```python
from build123d import *

# Parameters (mm, degrees)
SKETCH1_W                       = 9
SKETCH1_H                       = 18
SKETCH1_R                       = 1.9
BODY_MOUNT_DEPTH                = 3
SKETCH2_W                       = 5
SKETCH2_H                       = 3
BOSS_EXTRUDE2_DEPTH             = 25
SKETCH3_W                       = 5
SKETCH3_H                       = 5
BOSS_EXTRUDE3_DEPTH             = 20
SKETCH4_R                       = 1.5
CUT_EXTRUDE1_DEPTH              = 20
BOSS_EXTRUDE4_REACH             = 38.359
BOSS_EXTRUDE4_DIRECTION_2_REACH = 38.359
FILLET2_R                       = 5


with BuildPart() as part:
    # Sketch1 → body mount (new body)
    with BuildSketch(Plane(origin=(0, 0, 0), x_dir=(1, 0, 0), z_dir=(0, 1, 0))):
        with Locations((-0.5, 5)):
            Rectangle(SKETCH1_W, SKETCH1_H)
        with Locations(Location((0, 0, 0), (0, 0, 270))):
            Circle(SKETCH1_R, mode=Mode.SUBTRACT)
        with Locations(Location((0, 10, 0), (0, 0, 270))):
            Circle(SKETCH1_R, mode=Mode.SUBTRACT)
    extrude(amount=BODY_MOUNT_DEPTH)

    # Sketch2 → Boss-Extrude2 (add)
    with BuildSketch(Plane(origin=(4, 0, 0), x_dir=(0, 0, -1), z_dir=(1, 0, 0))):
        with Locations((5, 1.5)):
            Rectangle(SKETCH2_W, SKETCH2_H)
    extrude(amount=BOSS_EXTRUDE2_DEPTH)

    # Sketch3 → Boss-Extrude3 (add)
    with BuildSketch(Plane.XZ):
        with Locations((26.5, -5)):
            Rectangle(SKETCH3_W, SKETCH3_H)
    extrude(amount=BOSS_EXTRUDE3_DEPTH)

    # Sketch4 → Cut-Extrude1 (cut)
    with BuildSketch(Plane(origin=(0, 0, -7.5), x_dir=(-1, 0, 0), z_dir=(0, 0, -1))):
        with Locations((-26.5, -17)):
            Circle(SKETCH4_R)
        with Locations((-26.5, -7.5)):
            Circle(SKETCH4_R)
    extrude(amount=-CUT_EXTRUDE1_DEPTH, mode=Mode.SUBTRACT)

    # Boss-Extrude4: up to this face of the body (flat: up to its plane)
    boss_extrude4_end = Plane(part.part.faces().sort_by_distance((16.5, 2.660294245, -7.5))[0])
    # Sketch5 → Boss-Extrude4 (add, up to the picked face)
    with BuildSketch(Plane(origin=(0, 0, -5), x_dir=(-1, 0, 0), z_dir=(0, 0, -1)), mode=Mode.PRIVATE) as boss_extrude4_sk1:
        Polygon((-24, -10.415369352), (-9.210305315, 0), (-4, 0), (-24, -14.084630648), align=None)
    boss_extrude4_tool1 = split(extrude(boss_extrude4_sk1.sketch, amount=BOSS_EXTRUDE4_REACH, mode=Mode.PRIVATE), bisect_by=boss_extrude4_end, keep=Keep.BOTH, mode=Mode.PRIVATE)
    add(boss_extrude4_tool1.solids().sort_by(Axis((15.237549, -6.170794, -5), (0, 0, -1)))[0])

    # Boss-Extrude4 direction 2: up to this face of the body (flat: up to its plane)
    boss_extrude4_direction_2_end = Plane(part.part.faces().sort_by_distance((14, 0.339705755, -2.5))[0])
    # Sketch5 → Boss-Extrude4 direction 2 (add, up to the picked face)
    with BuildSketch(Plane(origin=(0, 0, -5), x_dir=(-1, 0, 0), z_dir=(0, 0, -1)), mode=Mode.PRIVATE) as boss_extrude4_direction_2_sk1:
        Polygon((-24, -10.415369352), (-9.210305315, 0), (-4, 0), (-24, -14.084630648), align=None)
    boss_extrude4_direction_2_tool1 = split(extrude(boss_extrude4_direction_2_sk1.sketch, amount=-BOSS_EXTRUDE4_DIRECTION_2_REACH, mode=Mode.PRIVATE), bisect_by=boss_extrude4_direction_2_end, keep=Keep.BOTH, mode=Mode.PRIVATE)
    add(boss_extrude4_direction_2_tool1.solids().sort_by(Axis((15.237549, -6.170794, -5), (0, 0, 1)))[0])

    # Fillet2
    # the kernel refuses this fillet: 5 mm, written as the material it adds along each edge
    with BuildSketch(Plane(origin=(4, 3, -7.5), x_dir=(0, 0, -1), z_dir=(0, -1, 0))) as fillet2_piece_1_section:
        with BuildLine():
            CenterArc((FILLET2_R, FILLET2_R), FILLET2_R, 180, 90)
            Line((0, FILLET2_R), (0, 0))
            Line((0, 0), (FILLET2_R, 0))
        make_face()
    fillet2_piece_1 = extrude(amount=3, mode=Mode.PRIVATE)
    fillet2_piece_1 = split(fillet2_piece_1, bisect_by=Plane(origin=(4.050655402, -0.035673131, -8.630736825), z_dir=(0.5757819971310116, 0.8176032606220598, 0)), keep=Keep.TOP, mode=Mode.PRIVATE)
    add(fillet2_piece_1)
    with BuildSketch(Plane(origin=(4, 3, -7.5), x_dir=(0, 0, -1), z_dir=(0, -1, 0))) as fillet2_piece_2_section:
        with BuildLine():
            CenterArc((FILLET2_R, FILLET2_R), FILLET2_R, 180, 90)
            Line((0, FILLET2_R), (0, 0))
            Line((0, 0), (FILLET2_R, 0))
        make_face()
    fillet2_piece_2 = extrude(amount=15.5, mode=Mode.PRIVATE)
    fillet2_piece_2 = split(fillet2_piece_2, bisect_by=Plane(origin=(6.150590259, 0, -8.032362576), z_dir=(0, -1, 0)), keep=Keep.TOP, mode=Mode.PRIVATE)
    fillet2_piece_2 = split(fillet2_piece_2, bisect_by=Plane(origin=(5.79410314, -1.263464003, -8.032362576), z_dir=(0.5757819971310116, 0.8176032606220598, 0)), keep=Keep.TOP, mode=Mode.PRIVATE)
    add(fillet2_piece_2)
    with BuildSketch(Plane(origin=(4, -12.5, -2.5), x_dir=(1, 0, 0), z_dir=(0, 1, 0))) as fillet2_piece_3_section:
        with BuildLine():
            CenterArc((FILLET2_R, -FILLET2_R), FILLET2_R, 90, 90)
            Line((0, -FILLET2_R), (0, 0))
            Line((0, 0), (FILLET2_R, 0))
        make_face()
    fillet2_piece_3 = extrude(amount=15.5, mode=Mode.PRIVATE)
    fillet2_piece_3 = split(fillet2_piece_3, bisect_by=Plane(origin=(5.79410314, -1.263464003, -1.967637424), z_dir=(0.5757819971310116, 0.8176032606220598, 0)), keep=Keep.TOP, mode=Mode.PRIVATE)
    fillet2_piece_3 = split(fillet2_piece_3, bisect_by=Plane(origin=(6.150590259, 0, -1.967637424), z_dir=(0, -1, 0)), keep=Keep.TOP, mode=Mode.PRIVATE)
    add(fillet2_piece_3)
    with BuildSketch(Plane(origin=(4, 0, -2.5), x_dir=(1, 0, 0), z_dir=(0, 1, 0))) as fillet2_piece_4_section:
        with BuildLine():
            CenterArc((FILLET2_R, -FILLET2_R), FILLET2_R, 90, 90)
            Line((0, -FILLET2_R), (0, 0))
            Line((0, 0), (FILLET2_R, 0))
        make_face()
    fillet2_piece_4 = extrude(amount=3, mode=Mode.PRIVATE)
    fillet2_piece_4 = split(fillet2_piece_4, bisect_by=Plane(origin=(4.050655402, -0.035673131, -1.369263175), z_dir=(0.5757819971310116, 0.8176032606220598, 0)), keep=Keep.TOP, mode=Mode.PRIVATE)
    add(fillet2_piece_4)


solid = part.part
```
CAD build for the part. Positions are in the model's coordinates, mm. A direction names the side the tool comes from. Coordinates: 2 decimals unless noted, no trailing zeros. Order: outer loops, then holes, each group sorted by start corner. A loop starts at its lowest first (then second) coordinate and runs counter-clockwise, first axis right, second up. Notation, with made-up numbers: M 43.5,28.5 L 88.5,28.5 A23 cw 88.5,45.5 Z; hole C 1.5,49 d3. An arc over 180 degrees is marked long. Answer as CSV lines item,"result".
1) Cut at A-A (x = 0). List the corners of the cut face in (y, z).
Verdict:
outline,"M 0,-14 L 3,-14 L 3,-11.9 L 0,-11.9 Z; M 0,-8.1 L 3,-8.1 L 3,-1.9 L 0,-1.9 Z; M 0,1.9 L 3,1.9 L 3,4 L 0,4 Z"
2) Flat gauge pins, fed straight in: P1, Ø1.2, axis at y = 1.5, z = -13, coming from the +X side; P2, Ø5, axis at x = 26.5, y = -17, coming from the -Z side; P3, Ø1.5, axis at y = -18.5, z = -6, coming from the -X side. Where does each tip first touch, or does it go through?
Verdict:
P1,"x = 4"
P2,"z = -7.5"
P3,"x = 24"
3) Mould opens along X. For faces 1 (the flat face through (26, -20, -5)), 2 (the cylindrical face through (6.18, 0.42, -1.63)), 3 (the flat face through (24, -5, -5)), 4 (the flat face through (24, -17, -5)) say: released by +X, released by -X, zero draft, split by the parting line, or undercut.
Verdict:
face 1,"zero draft"
face 2,"released by +X"
face 3,"undercut"
face 4,"released by -X"
4) Cut at B-B (y = -17). List the corners of the cut face in (x, z), then the cut area to 3 significant figures.
Verdict:
outline,"M 24,-7.5 L 25,-7.5 L 25,-2.5 L 24,-2.5 Z; M 28,-7.5 L 29,-7.5 L 29,-2.5 L 28,-2.5 Z"
area,"10.0 mm2"
5) 3-axis set-ups, long thin cutter, end or side, ignore diameter. For faces 5 (the flat face through (4, 1, 3)), 6 (the flat face through (8, 3, -5)), 7 (the flat face through (21, -9, -7.5)), 8 (the flat face through (17, 0, -5)), 9 (the flat face through (-5, 1, -5)): which of +Z, -Z, +X, -X, +Y, -Y reach the whole face in a straight line?
Verdict:
face 5,"+Z, +X, +Y, -Y"
face 6,"+Z, -Z, +X, -X, +Y"
face 7,"-Z, +X, +Y, -Y"
face 8,"+Z, -Z"
face 9,"+Z, -Z, -X, +Y, -Y"
6) Cut at D-D (y = 1). List the corners of the cut face in (x, z).
Verdict:
outline,"M -5,-14 L 4,-14 L 4,-12.5 A5 cw 9,-7.5 L 29,-7.5 L 29,-2.5 L 9,-2.5 A5 cw 4,2.5 L 4,4 L -5,4 Z; hole C 0,-10 d3.8; hole C 0,0 d3.8"
7) Drill centre lines: L1, parallel to Y at x = 26.5, z = -4.6; L2, parallel to Y at x = 0, z = -6; L3, parallel to X at y = 1.65, z = -10. Where is each one in solid material? Low to high. Write a range as from..to.
Verdict:
L1,"-20..-18.5, -15.5..-9, -6..3"
L2,"0..3"
L3,"-5..-1.9, 1.9..4.67"
8) Cut at C-C (z = 0). List the corners of the cut face in (x, y), then the cut area to 3 significant figures.
Verdict:
outline,"M -5,0 L -1.9,0 L -1.9,3 L -5,3 Z; M 1.9,0 L 4,0 L 4.67,-0.47 L 4.67,3 L 1.9,3 Z"
area,"17.8 mm2"
